Print and shaded views of the part. All mm, measured from the part's lowest x, y and z. A direction names the side the tool comes from. Round coordinates to 2 decimals unless told otherwise and drop trailing zeros. Write each loop counter-clockwise with the first axis right and the second up, starting at its lowest first coordinate (ties: lowest second). Pieces come first, ordered by that corner, then holes. Notation, with made-up numbers: (-7.75, 75.25) - (-2.75, 75.25) arc R5 cw to (-2.75, 83.25) - close; hole circle Ø9 at (85.5, -35). An arc over 180 degrees is marked (long way). One line per item, written item: value.
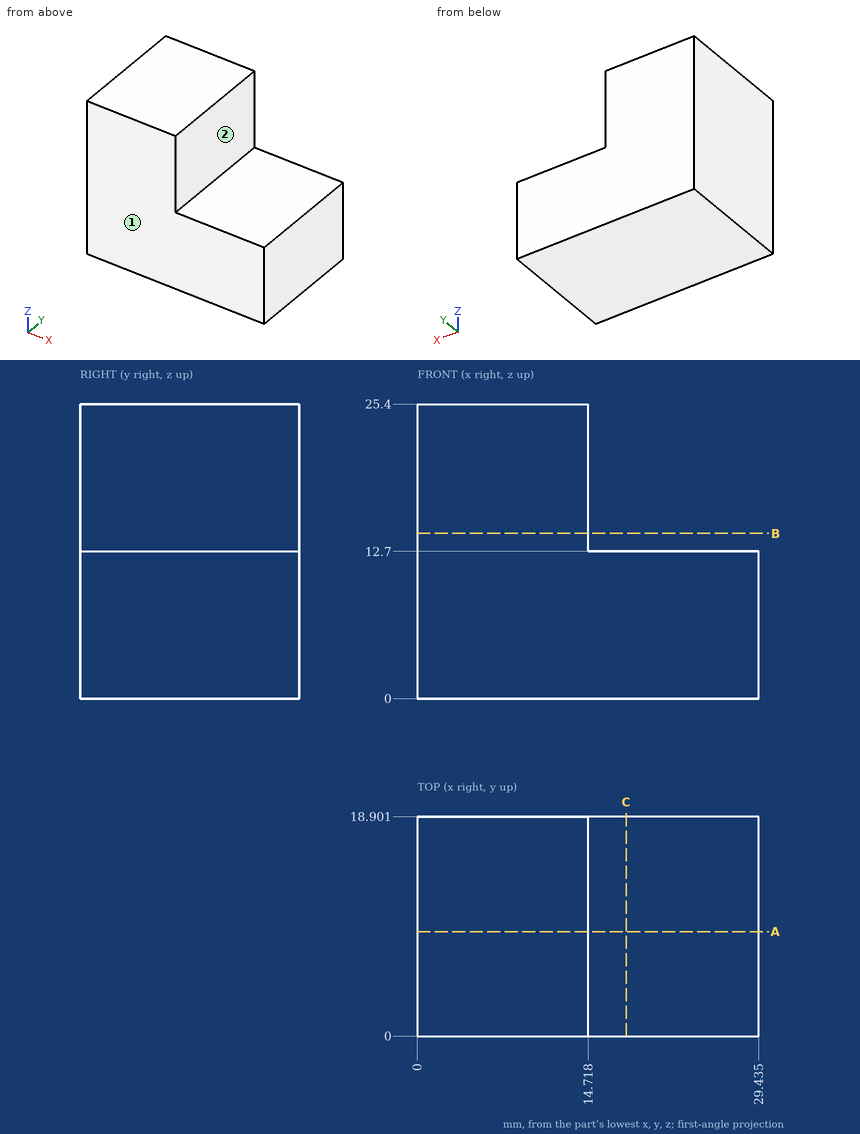
1. Band-saw the part on B-B on z = 14.25. Write the cut outline in (x, y), plus the area to 3 significant figures.
Report:
outline: (0, 0) - (14.72, 0) - (14.72, 18.9) - (0, 18.9) - close
area: 278 mm²
2. Band-saw the part on A-A on y = 9. Write the cut outline in (x, z) (1 decimal).
Report:
outline: (0, 0) - (29.4, 0) - (29.4, 12.7) - (14.7, 12.7) - (14.7, 25.4) - (0, 25.4) - close
3. Drop flat-ended pins along their axis: pin 1 (2 mm diameter, centred on x = 20.5, y = 13, fed in from +Z); pin 2 (1.5 mm diameter, centred on y = 13, z = 16.5, fed in from +X). Give the stop position or say it passes through.
Report:
pin 1: z = 12.7
pin 2: x = 14.72
4. Wall check: probe 1 along X at (y, z) = (2.5, 22.75); probe 2 along Z at (x, y) = (24.25, 13.25). Give the ranges that are in metal, low to high. Write a range as [from, to].
Report:
probe 1: [0, 14.72]
probe 2: [0, 12.7]
5. Band-saw the part on C-C on x = 18. Write the cut outline in (y, z).
Report:
outline: (0, 0) - (18.9, 0) - (18.9, 12.7) - (0, 12.7) - close
6. Tool access for the marked faces 1 and 2: list every direction of +Z, -Z, +X, -X, +Y, -Y with a clear straight run to the whole face (end or side of a thin tool).
Report:
face 1: +Z, -Z, +X, -X, -Y
face 2: +Z, +X, +Y, -Y
